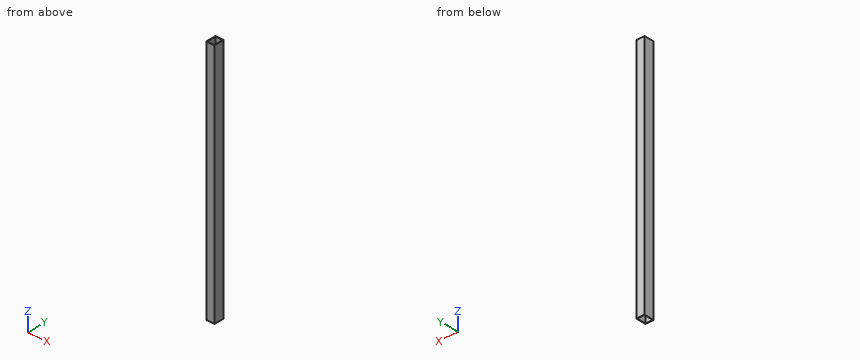
```python
from build123d import *

# Parameters (mm, degrees)
SKETCH4_W           = 1219.2
SKETCH4_H           = 50.8
BOSS_EXTRUDE2_DEPTH = 41.275
SHELL7_T            = -2.54


with BuildPart() as part:
    # Sketch4 → Boss-Extrude2 (new body)
    with BuildSketch(Plane(origin=(0, 0, 0), x_dir=(0, 0, -1), z_dir=(1, 0, 0))):
        with Locations((275.6, -77.4)):
            Rectangle(SKETCH4_W, SKETCH4_H)
    extrude(amount=-BOSS_EXTRUDE2_DEPTH)

    # Shell7
    shell7_openings = [part.faces().sort_by_distance(p)[0] for p in [
        (-20.6375, -77.4, -885.2),
        (-20.6375, -77.4, 334),
    ]]
    offset(amount=SHELL7_T, openings=shell7_openings, kind=Kind.INTERSECTION)


solid = part.part
```
Check sheet for the modelled part. Datum: model origin and axes. Units: mm. Round coordinates to 2 decimals unless told otherwise and drop trailing zeros. Order: outer loops, then holes, each group sorted by start corner. A loop starts at its lowest first (then second) coordinate and runs counter-clockwise, first axis right, second up. Notation, with made-up numbers: (76.25, -16.75) -> (91.25, -16.75) arc R20 ccw to (91.25, 21.25) -> close; hole circle Ø8 at (-27.75, -8). An arc over 180 degrees is marked (long way). One line per item, written item: value. Start each with the question number.
Q1. Cross-section at C-C (z = 166). Record the boundary of the cut face in (x, y) (3 decimals), and give its area (3 significant figures).
Q2. Thickness scan on line 1 (X direction, y = -58, z = -746.5) (3 decimals); line 2 (Y direction, x = -30, z = 28.5). Record the ranges inside material, lowest first.
Q3. Cross-section at B-B (x = -13.5). Record the boundary of the cut face in (y, z), and give its area (3 significant figures).
Q4. Cross-section at A-A (y = -91.5). Record the boundary of the cut face in (x, z) (3 decimals), and give its area (3 significant figures).
Q5. Gauge pin test, flat ends, axial feed: pin 1 Ø4 at (y, z) = (-70.5, -533) entering from +X; pin 2 Ø12 at (x, y) = (-28.5, -79.5) entering from +Z. Record the tip position at first contact, or that the pin passes through.
Completed:
1. outline: (-41.275, -102.8) -> (0, -102.8) -> (0, -52) -> (-41.275, -52) -> close; hole (-38.735, -100.26) -> (-2.54, -100.26) -> (-2.54, -54.54) -> (-38.735, -54.54) -> close
1. area: 442 mm²
2. line 1: x = -41.275 to -38.735, -2.54 to 0
2. line 2: y = -102.8 to -100.26, -54.54 to -52
3. outline: (-102.8, -885.2) -> (-100.26, -885.2) -> (-100.26, 334) -> (-102.8, 334) -> close; (-54.54, -885.2) -> (-52, -885.2) -> (-52, 334) -> (-54.54, 334) -> close
3. area: 6,190 mm²
4. outline: (-41.275, -885.2) -> (-38.735, -885.2) -> (-38.735, 334) -> (-41.275, 334) -> close; (-2.54, -885.2) -> (0, -885.2) -> (0, 334) -> (-2.54, 334) -> close
4. area: 6,190 mm²
5. pin 1: stops at x = 0
5. pin 2: passes through
